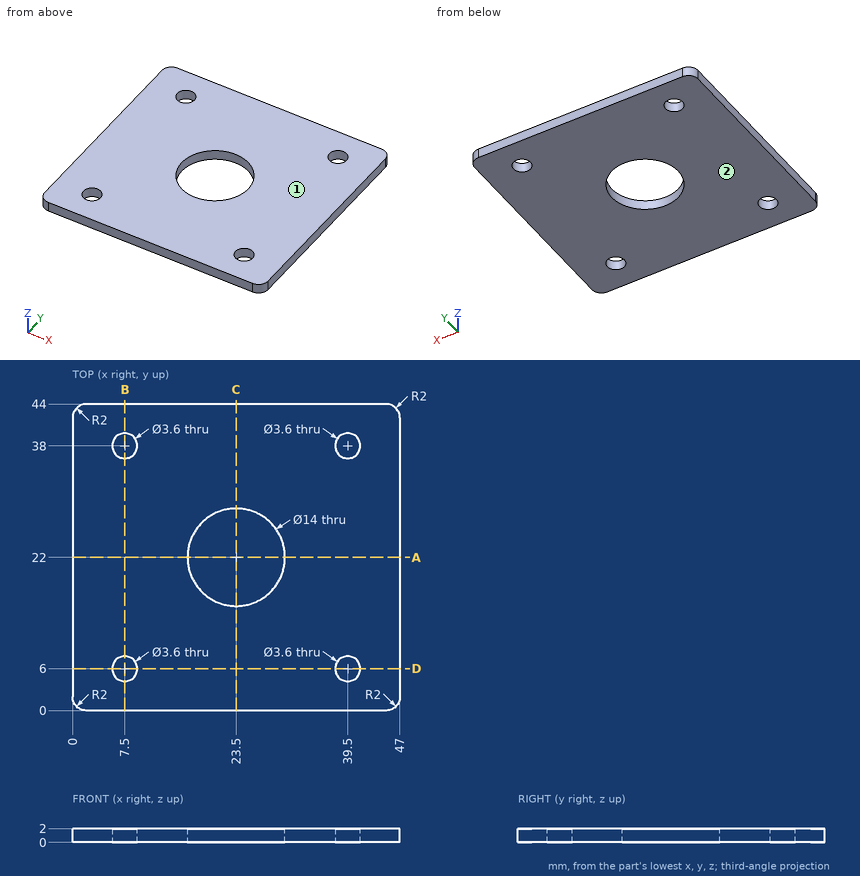
Input: dimensioned drawing with shaded views. Units: mm. Origin: part minimum x, y, z. Coordinates: 2 decimals unless noted, no trailing zeros. Loops run counter-clockwise (first coordinate to the right, second up) from the corner with the lowest first, then second, coordinate; pieces in that order, holes last. Notation, with made-up numbers: M -40,-9 L -18,-9 A13 ccw -18,14 Z; hole C -9,67.25 d4. An arc over 180 degrees is marked long. Use a Markdown table: item, result. Add a question column.
Q1. Section query D-D, the plane y = 6. Return loops of the section in (x, z).
Q2. Draft query along Z for the marked faces 1 and 2. Return one class per face: pulls with the +Z half, pulls with the -Z half, needs draft (parallel to the pull), parting line crosses it, or undercut.
Q3. Section query A-A, the plane y = 22. Return loops of the section in (x, z).
Q4. Section query B-B, the plane x = 7.5. Return loops of the section in (y, z), and give its area (3 significant figures).
Q5. Section query C-C, the plane x = 23.5. Return loops of the section in (y, z), and give its area (3 significant figures).
Q6. Material intervals for L1, parallel to Y at x = 39.5, z = 0.7; L2, parallel to Y at x = 23.5, z = 1.1; L3, parallel to Y at x = 7, z = 1.8, sorted ascending.
Result:
| question | item | result |
|---|---|---|
| 1 | outline | M 0,0 L 5.7,0 L 5.7,2 L 0,2 Z; M 9.3,0 L 37.7,0 L 37.7,2 L 9.3,2 Z; M 41.3,0 L 47,0 L 47,2 L 41.3,2 Z |
| 2 | face 1 | pulls with the +Z half |
| 2 | face 2 | pulls with the -Z half |
| 3 | outline | M 0,0 L 16.5,0 L 16.5,2 L 0,2 Z; M 30.5,0 L 47,0 L 47,2 L 30.5,2 Z |
| 4 | outline | M 0,0 L 4.2,0 L 4.2,2 L 0,2 Z; M 7.8,0 L 36.2,0 L 36.2,2 L 7.8,2 Z; M 39.8,0 L 44,0 L 44,2 L 39.8,2 Z |
| 4 | area | 73.6 mm2 |
| 5 | outline | M 0,0 L 15,0 L 15,2 L 0,2 Z; M 29,0 L 44,0 L 44,2 L 29,2 Z |
| 5 | area | 60.0 mm2 |
| 6 | L1 | y = 0 to 4.2, 7.8 to 36.2, 39.8 to 44 |
| 6 | L2 | y = 0 to 15, 29 to 44 |
| 6 | L3 | y = 0 to 4.27, 7.73 to 36.27, 39.73 to 44 |
